from build123d import *

# Parameters (mm, degrees)
SKETCH1_W           = 39.878
SKETCH1_H           = 24
BOSS_EXTRUDE1_DEPTH = 9
SKETCH2_W           = 28
SKETCH2_H           = 16
CUT_EXTRUDE1_DEPTH  = 25.951226844
SKETCH4_R           = 1.5
CUT_EXTRUDE2_DEPTH  = 25.951226844


with BuildPart() as part:
    # Sketch1 → Boss-Extrude1 (new body)
    with BuildSketch(Plane(origin=(0, 0, 0), x_dir=(1, 0, 0), z_dir=(0, 1, 0))):
        Rectangle(SKETCH1_W, SKETCH1_H)
    extrude(amount=BOSS_EXTRUDE1_DEPTH)

    # Sketch2 → Cut-Extrude1 (cut, through all)
    with BuildSketch(Plane(origin=(0, 9, 0), x_dir=(1, 0, 0), z_dir=(0, 1, 0))):
        with Locations((5.939, -4)):
            Rectangle(SKETCH2_W, SKETCH2_H)
    extrude(amount=-CUT_EXTRUDE1_DEPTH, mode=Mode.SUBTRACT)

    # Sketch4 → Cut-Extrude2 (cut, through all)
    with BuildSketch(Plane(origin=(0, 9, 0), x_dir=(1, 0, 0), z_dir=(0, 1, 0))):
        with Locations(Location((-12.589, -8.509, 0), (0, 0, 270))):
            Circle(SKETCH4_R)
        with Locations(Location((-12.589, 8.509, 0), (0, 0, 270))):
            Circle(SKETCH4_R)
    extrude(amount=-CUT_EXTRUDE2_DEPTH, mode=Mode.SUBTRACT)


solid = part.part
Input: part model. Units: mm. Frame: model coordinates. A direction names the side the tool comes from. Give positions to 0.01 mm unless a question says otherwise; leave off trailing zeros. Write each loop counter-clockwise with the first axis right and the second up, starting at its lowest first coordinate (ties: lowest second). Pieces come first, ordered by that corner, then holes.
Q1. Pull-direction query (X, two-part tool) for faces 3 (the face through (19.939, 4, -8)), 4 (the face through (-12.523, 4.563, -10.008)), 5 (the face through (-11.324, 4.563, 9.315)), 6 (the face through (-5, 9, -6)); classes: pulls with the +X half, pulls with the -X half, needs draft (parallel to the pull), parting line crosses it, or undercut.
Q2. Material intervals for probe 1 along Z at (x, y) = (-7.5, 3.5); probe 2 along X at (y, z) = (1.25, -3.75); probe 3 along X at (y, z) = (5.5, 7.75), sorted ascending.
Q3. Section D-D, the plane z = 2. Output: boundary loops of the cut face in (x, y), plus the area to 3 significant figures.
Q4. Set-up query: faces 1 (the face through (0, 4, -12)), 2 (the face through (6, 5, -4)). Return all of +Z, -Z, +X, -X, +Y, -Y with unobstructed straight access to the full face (end or side cutting, diameter ignored); none if empty.
Q5. Section C-C, the plane x = 7. Output: boundary loops of the cut face in (y, z), plus the area to 3 significant figures.
Q6. Section B-B, the plane y = 8. Output: boundary loops of the cut face in (x, z), plus the area to 3 significant figures.
Q7. Section A-A, the plane z = 9.5. Output: boundary loops of the cut face in (x, y).
Q8. First-contact query: P1, Ø4, axis at y = 4.5, z = 6.5, coming from the +X side; P2, Ø4.5, axis at x = 3.5, y = 6.5, coming from the +Z side. Flat tips, straight axial feed; report the tip coordinate or a pass-through.
Filled in:
1. face 3: pulls with the +X half
1. face 4: undercut
1. face 5: undercut
1. face 6: needs draft
2. probe 1: z = -12 to -4
2. probe 2: x = -19.94 to -8.06
2. probe 3: x = -19.94 to -13.88, -11.3 to -8.06
3. outline: (-19.94, 0) - (-8.06, 0) - (-8.06, 9) - (-19.94, 9) - close
3. area: 107 mm2
4. face 1: -Z, +X, -X, +Y, -Y
4. face 2: +Z, +X, +Y, -Y
5. outline: (0, -12) - (9, -12) - (9, -4) - (0, -4) - close
5. area: 72.0 mm2
6. outline: (-19.94, -12) - (19.94, -12) - (19.94, -4) - (-8.06, -4) - (-8.06, 12) - (-19.94, 12) - close; hole circle Ø3 at (-12.59, -8.51); hole circle Ø3 at (-12.59, 8.51)
6. area: 495 mm2
7. outline: (-19.94, 0) - (-13.72, 0) - (-13.72, 9) - (-19.94, 9) - close; (-11.46, 0) - (-8.06, 0) - (-8.06, 9) - (-11.46, 9) - close
8. P1: stops at x = -8.06
8. P2: stops at z = -4
